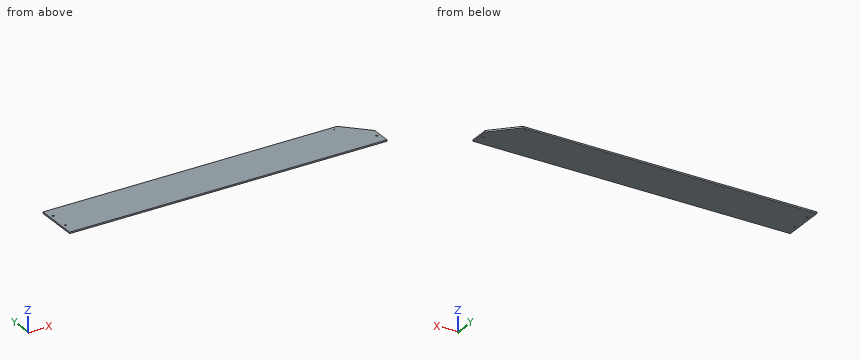
```python
from build123d import *

# Parameters (mm, degrees)
BOSS_EXTRUDE1_DEPTH = 4
SKETCH8_R           = 2.6
CUT_EXTRUDE4_DEPTH  = 10
SKETCH9_R           = 2.6
CUT_EXTRUDE5_DEPTH  = 10
SKETCH10_R          = 1.5
CUT_EXTRUDE6_DEPTH  = 894.10749633


with BuildPart() as part:
    # Sketch1 → Boss-Extrude1 (new body)
    with BuildSketch(Plane.XY):
        Polygon((0, 0), (885, 0), (885, 55), (820, 120), (0, 120), align=None)
    extrude(amount=BOSS_EXTRUDE1_DEPTH)


with BuildPart() as part_1:
    # Body-Move/Copy1: moved
    add(part.part.moved(Location((0, 0, -4))))

    # Sketch8 → Cut-Extrude4 (cut)
    with BuildSketch(Plane.XY):
        with Locations((10, 90)):
            Circle(SKETCH8_R)
        with Locations((10, 35)):
            Circle(SKETCH8_R)
    extrude(amount=-CUT_EXTRUDE4_DEPTH, mode=Mode.SUBTRACT)

    # Sketch9 → Cut-Extrude5 (cut)
    with BuildSketch(Plane.XY):
        with Locations((875, 30)):
            Circle(SKETCH9_R)
    extrude(amount=-CUT_EXTRUDE5_DEPTH, mode=Mode.SUBTRACT)

    # Sketch10 → Cut-Extrude6 (cut, through all)
    with BuildSketch(Plane.XY):
        with Locations((806, 110)):
            Circle(SKETCH10_R)
    extrude(amount=-CUT_EXTRUDE6_DEPTH, mode=Mode.SUBTRACT)


solid = part_1.part
```
Here's how the part is built. I have some questions about the finished solid (model axes, mm). Give positions to 0.01 mm unless a question says otherwise; leave off trailing zeros. Order: outer loops, then holes, each group sorted by start corner. A loop starts at its lowest first (then second) coordinate and runs counter-clockwise, first axis right, second up. Notation, with made-up numbers: M -1.5,-13.5 L 21.5,-13.5 A34 ccw 21.5,23.5 Z; hole C 0,80.25 d9. An arc over 180 degrees is marked long. Use a Markdown table: item, result. Add a question column.
1. Suppose I cut it at A-A (z = -0.6). List the corners of the cut face in (x, y) for me, and give its area (3 significant figures).
2. For pin 1 Ø4.5 at (x, y) = (875, 30) entering from +Z, with a flat end and sliding along its axis, tell me the tip position at first contact or that it passes through.
3. I need wall thicknesses on probe 1 along X at (y, z) = (110, -0.9); probe 2 along X at (y, z) = (33, -0.9); probe 3 along Y at (x, z) = (875, -1.8). Which ranges of each line are inside material? Lowest first, please. Write a range as from..to.
Results list:
| question | item | result |
|---|---|---|
| 1 | outline | M 0,0 L 885,0 L 885,55 L 820,120 L 0,120 Z; hole C 10,35 d5.2; hole C 10,90 d5.2; hole C 806,110 d3; hole C 875,30 d5.2 |
| 1 | area | 104,000 mm² |
| 2 | pin 1 | passes through |
| 3 | probe 1 | x = 0..804.5, 807.5..830 |
| 3 | probe 2 | x = 0..8.34, 11.66..885 |
| 3 | probe 3 | y = 0..27.4, 32.6..65 |
